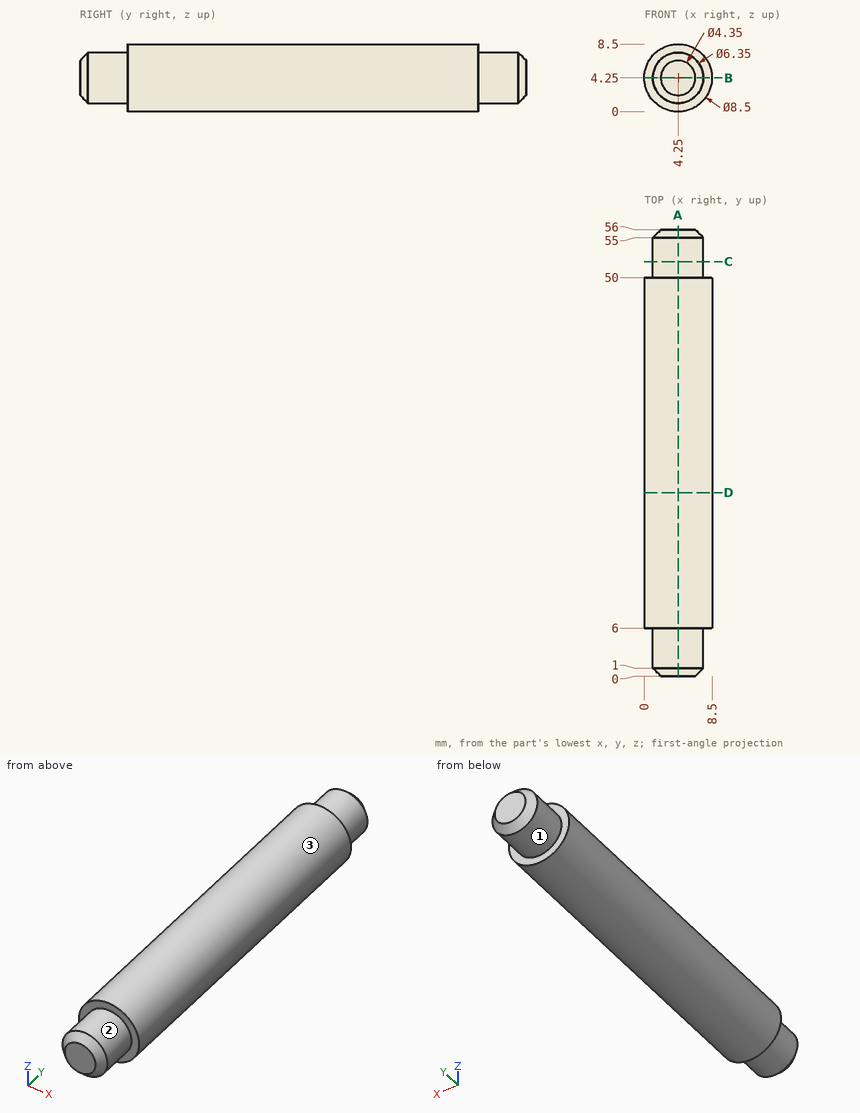
Geometry: see drawing. Coordinates: mm, zero at the bounding-box minimum. A direction names the side the tool comes from. Give positions to 0.01 mm unless a question says otherwise; leave off trailing zeros. Order: outer loops, then holes, each group sorted by start corner. A loop starts at its lowest first (then second) coordinate and runs counter-clockwise, first axis right, second up. Notation, with made-up numbers: (-15.5, 45) -> (13.5, 45) arc R9 ccw to (13.5, 57) -> close; hole circle Ø10 at (86.25, 81). An arc over 180 degrees is marked (long way). Write item = value, one per line.
Q1. Set-up query: the marked faces 1, 2 and 3. Return all of +Z, -Z, +X, -X, +Y, -Y with unobstructed straight access to the full face (end or side cutting, diameter ignored); none if empty.
Data:
face_1 = +Y
face_2 = -Y
face_3 = +Y, -Y
Q2. Cut plane C-C, the plane y = 52. Output: boundary loops of the cut face in (x, z) (3 decimals), and give its area (3 significant figures).
Data:
outline = circle Ø6.35 at (4.25, 4.25)
area = 31.7 mm^2
Q3. Material intervals for line 1 (Y direction, x = 8, z = 3.75); line 2 (Z direction, x = 4, y = 11); line 3 (Z direction, x = 6.5, y = 33.5), sorted ascending. Write a range as from..to.
Data:
line_1 = 6..50
line_2 = 0.01..8.49
line_3 = 0.64..7.86
Q4. Cut plane A-A, the plane x = 4.25. Output: boundary loops of the cut face in (y, z) (3 decimals).
Data:
outline = (0, 2.075) -> (1, 1.075) -> (6, 1.075) -> (6, 0) -> (50, 0) -> (50, 1.075) -> (55, 1.075) -> (56, 2.075) -> (56, 6.425) -> (55, 7.425) -> (50, 7.425) -> (50, 8.5) -> (6, 8.5) -> (6, 7.425) -> (1, 7.425) -> (0, 6.425) -> close
Q5. Cut plane D-D, the plane y = 23. Output: boundary loops of the cut face in (x, z), and give its area (3 significant figures).
Data:
outline = circle Ø8.5 at (4.25, 4.25)
area = 56.7 mm^2
Q6. Cut plane B-B, the plane z = 4.25. Output: boundary loops of the cut face in (x, y) (3 decimals).
Data:
outline = (0, 6) -> (1.075, 6) -> (1.075, 1) -> (2.075, 0) -> (6.425, 0) -> (7.425, 1) -> (7.425, 6) -> (8.5, 6) -> (8.5, 50) -> (7.425, 50) -> (7.425, 55) -> (6.425, 56) -> (2.075, 56) -> (1.075, 55) -> (1.075, 50) -> (0, 50) -> close
Q7. Pin query (flat end, axial travel): pin 1 (1.5 mm diameter, centred on x = 5, y = 44, fed in from -Z); pin 2 (1.5 mm diameter, centred on x = 1, y = 43.5, fed in from -Z); pin 3 (1.5 mm diameter, centred on y = 17.5, z = 1.5, fed in from -X); pin 4 (3 mm diameter, centred on x = 6.5, y = 40.5, fed in from +Z). Return the tip coordinate at first contact, or that it passes through.
Data:
pin_1 = 0
pin_2 = 0.81
pin_3 = 0.5
pin_4 = 8.43
